```python
from build123d import *

# Parameters (mm, degrees)
F1_DEPTH = 63.5
F2_DEPTH = 38.1
F4_R     = 5.08
F5_R     = 5.08


with BuildPart() as f1:
    # F0 (on Front) → F1 (new body, symmetric)
    with BuildSketch(Plane.XZ):
        Polygon((-41.275, -9.525), (41.275, -9.525), (41.275, 9.525), (22.225, 9.525), (-41.275, 9.525), align=None)
    extrude(amount=F1_DEPTH, both=True)

    # F0 (on Front) → F2 (join, symmetric)
    with BuildSketch(Plane.XZ):
        with BuildLine():
            Line((22.225, 9.525), (41.275, 9.525))
            Line((41.275, 9.525), (41.275, 26.1178162626))
            ThreePointArc((41.275, 26.1178162626), (45.9246798487, 37.3431364139), (57.15, 41.9928162626))
            Line((57.15, 41.9928162626), (60.325, 41.9928162626))
            Line((60.325, 41.9928162626), (60.325, 61.0428162626))
            Line((60.325, 61.0428162626), (57.15, 61.0428162626))
            add(Edge.make_bspline(
                [(53.270143605, 60.8266384747), (54.5515105063, 60.9068312899), (55.8448088672, 60.9788851621), (57.15, 61.0428162626)],
                knots=[108.4277797835, 108.4277797835, 108.4277797835, 108.4277797835, 111.0926010924, 111.0926010924, 111.0926010924, 111.0926010924], degree=3))
            ThreePointArc((53.270143605, 60.8266384747), (31.1186764686, 49.4014117796), (22.225, 26.1178162626))
            Line((22.225, 26.1178162626), (22.225, 9.525))
        make_face()
        Polygon((60.325, 61.0428162626), (60.325, 41.9928162626), (60.325, 41.9873446226), (85.725, 41.9873446226), (85.725, 42.3024737561), (85.725, 51.9704466166), (85.725, 52.3875), (85.725, 61.0428162626), align=None)
    extrude(amount=F2_DEPTH, both=True)

    # F0 (on Front) → F3 (revolve)
    with BuildSketch(Plane.XZ):
        Polygon((85.725, 66.675), (85.725, 61.0428162626), (85.725, 52.3875), (85.725, 51.9704466166), (85.725, 42.3024737561), (85.725, 41.9873446226), (85.725, 38.1), (111.125, 38.1), (111.125, 66.675), align=None)
    revolve(axis=Axis((85.725, 0, 56.7151581313), (0, 0, -1)))

    # F4
    f4_edges = [f1.edges().sort_by_distance(p)[0] for p in [
        (41.275, -63.5, 0),
    ]]
    fillet(f4_edges, radius=F4_R)

    # F5
    f5_edges = [f1.edges().sort_by_distance(p)[0] for p in [
        (-41.275, 63.5, 0),
        (-41.275, -63.5, 0),
        (41.275, 63.5, 0),
    ]]
    fillet(f5_edges, radius=F5_R)


solid = f1.part
```
Geometry check sheet. Reference: the model listing, model coordinates, mm. A direction names the side the tool comes from. Round coordinates to 2 decimals unless told otherwise and drop trailing zeros. Loops run counter-clockwise (first coordinate to the right, second up) from the corner with the lowest first, then second, coordinate; pieces in that order, holes last. Notation, with made-up numbers: (80, 3.25) -> (138, 3.25) arc R26 ccw to (138, 29.25) -> close; hole circle Ø9 at (14.5, 22.5). An arc over 180 degrees is marked (long way). Use a Markdown table: item, result.
(1) Go/stop test with flat-tipped pins: P1, Ø13.5, axis at y = -11, z = 21.5, coming from the -X side (3 decimals); P2, Ø8, axis at x = 80, y = 21, coming from the -Z side; P3, Ø6, axis at x = 34.5, z = 45, coming from the +Y side; P4, Ø5, axis at x = -4.5, z = 11, coming from the +Y side. Record where each tip stops, or that it passes through.
Calculated:
| item | result |
|---|---|
| P1 | x = 22.225 |
| P2 | z = 38.1 |
| P3 | y = 38.1 |
| P4 | y = 63.5 |
(2) Set-up check for faces 4 (the flat face through (85.725, 32, 51)), 5 (the flat face through (46, -38.1, 41)), 6 (the flat face through (22.225, -1, 18)): record each of +Z, -Z, +X, -X, +Y, -Y from which the full face is reachable in a straight line by a thin tool's end or side.
Calculated:
| item | result |
|---|---|
| face 4 | +Z, -Z, +X, +Y |
| face 5 | +Z, +X, -X, -Y |
| face 6 | +Z, -X, +Y, -Y |
(3) Mould release check, pull along X, two halves, no side actions. Record for faces 1 (the flat face through (-1, -63.5, 0)), 2 (the cylindrical face through (-39.75, 62.05, -0.13)), 3 (the flat face through (70, -28, 41.987)): released by +X, released by -X, zero draft, split by the parting line, or undercut.
Calculated:
| item | result |
|---|---|
| face 1 | zero draft |
| face 2 | released by -X |
| face 3 | undercut |
(4) Scan lines: probe 1 along X at (y, z) = (-26, 9) (3 decimals); probe 2 along Y at (x, z) = (25, 25); probe 3 along Z at (x, y) = (67, -27.5). Record each from-to range of solid material in increasing order.
Calculated:
| item | result |
|---|---|
| probe 1 | -41.275 to 41.275 |
| probe 2 | -38.1 to 38.1 |
| probe 3 | 41.99 to 61.04 |
(5) Sectioned sample at A-A (z = 3). Enter the section's corners in (x, y) (3 decimals), then the cut area to 3 significant figures.
Calculated:
| item | result |
|---|---|
| outline | (-41.275, -58.42) arc R5.08 ccw to (-36.195, -63.5) -> (36.195, -63.5) arc R5.08 ccw to (41.275, -58.42) -> (41.275, 58.42) arc R5.08 ccw to (36.195, 63.5) -> (-36.195, 63.5) arc R5.08 ccw to (-41.275, 58.42) -> close |
| area | 10,500 mm² |
(6) Sectioned sample at C-C (x = 7). Enter the section's corners in (y, z) (3 decimals).
Calculated:
| item | result |
|---|---|
| outline | (-63.5, -9.525) -> (63.5, -9.525) -> (63.5, 9.525) -> (-63.5, 9.525) -> close |
(7) Sectioned sample at D-D (x = 72). Enter the section's corners in (y, z) (3 decimals).
Calculated:
| item | result |
|---|---|
| outline | (-38.1, 41.987) -> (-21.373, 41.987) -> (-21.373, 38.1) -> (21.373, 38.1) -> (21.373, 41.987) -> (38.1, 41.987) -> (38.1, 61.043) -> (21.373, 61.043) -> (21.373, 66.675) -> (-21.373, 66.675) -> (-21.373, 61.043) -> (-38.1, 61.043) -> close |
(8) Sectioned sample at B-B (y = 41.5). Enter the section's corners in (x, z) (3 decimals).
Calculated:
| item | result |
|---|---|
| outline | (-41.275, -9.525) -> (41.275, -9.525) -> (41.275, 9.525) -> (-41.275, 9.525) -> close |
